from build123d import *

# Parameters (mm, degrees)
BOSS_EXTRUDE1_DEPTH            = 15
SKETCH11_W                     = 2.25
SKETCH11_H                     = 12.7
M4_CLEARANCE_HOLE5_AT_2_COUNT  = 2
M4_CLEARANCE_HOLE5_AT_2_PITCH  = 35
SKETCH13_W                     = 3.75
SKETCH13_H                     = 29.3
F_6_0MM_DOWEL_HOLE1_AT_2_COUNT = 2
F_6_0MM_DOWEL_HOLE1_AT_2_PITCH = 35
FILLET1_R                      = 6.35


with BuildPart() as part:
    # Sketch1 → Boss-Extrude1 (new body)
    with BuildSketch(Plane(origin=(0, 0, 0), x_dir=(1, 0, 0), z_dir=(0, 1, 0))):
        Polygon((0, 0), (0, 42), (22, 20), (44, 42), (44, 0), align=None)
    extrude(amount=BOSS_EXTRUDE1_DEPTH)

    # Sketch11 → M4 Clearance Hole5 (revolve, cut)
    with BuildSketch(Plane(origin=(39.5, 7.5, -12.7), x_dir=(0, 1, 0), z_dir=(1, 0, 0))):
        with Locations((1.125, 6.35)):
            Rectangle(SKETCH11_W, SKETCH11_H)
    m4_clearance_hole5 = revolve(axis=Axis((39.5, 7.5, -19.05), (0, 0, 1)), mode=Mode.SUBTRACT)

    # M4 Clearance Hole5 at 2: M4 Clearance Hole5 ×2
    with Locations(*[(-i * M4_CLEARANCE_HOLE5_AT_2_PITCH, 0, 0) for i in range(1, M4_CLEARANCE_HOLE5_AT_2_COUNT)]):
        add(m4_clearance_hole5, mode=Mode.SUBTRACT)

    # Sketch13 → Ø6.0mm Dowel Hole1 (revolve, cut)
    with BuildSketch(Plane(origin=(39.5, 7.5, -12.7), x_dir=(0, -1, 0), z_dir=(1, 0, 0))):
        with Locations((1.875, 14.65)):
            Rectangle(SKETCH13_W, SKETCH13_H)
    f_6_0mm_dowel_hole1 = revolve(axis=Axis((39.5, 7.5, -6.35), (0, 0, -1)), mode=Mode.SUBTRACT)

    # Ø6.0mm Dowel Hole1 at 2: Ø6.0mm Dowel Hole1 ×2
    with Locations(*[(-i * F_6_0MM_DOWEL_HOLE1_AT_2_PITCH, 0, 0) for i in range(1, F_6_0MM_DOWEL_HOLE1_AT_2_COUNT)]):
        add(f_6_0mm_dowel_hole1, mode=Mode.SUBTRACT)

    # Fillet1
    fillet1_edges = [part.edges().sort_by_distance(p)[0] for p in [
        (22, 7.5, -20),
    ]]
    fillet(fillet1_edges, radius=FILLET1_R)


solid = part.part
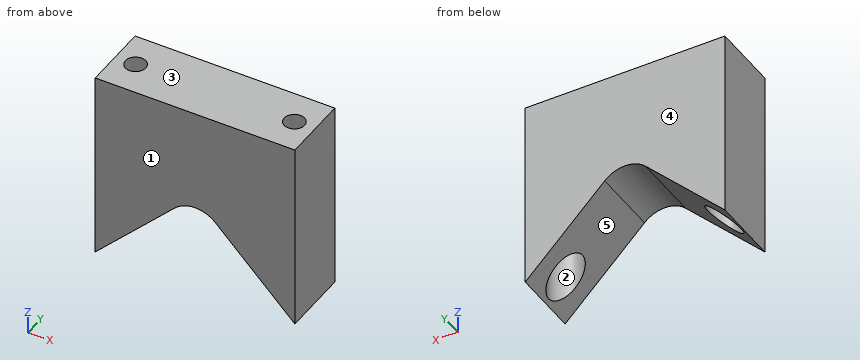
Verification items for the finished model (mm, model axes). Face numbers are marked on the shaded views. A direction names the side the tool comes from. Coordinates: 2 decimals unless noted, no trailing zeros. Write each loop counter-clockwise with the first axis right and the second up, starting at its lowest first coordinate (ties: lowest second). Pieces come first, ordered by that corner, then holes. Notation, with made-up numbers: (42.5, 68.5) -> (98.5, 68.5) arc R16 ccw to (98.5, 86.5) -> close; hole circle Ø9 at (60.5, 80). An arc over 180 degrees is marked (long way). One line per item, written item: value. Start each with the question number.
Q1. Thickness scan on L1, parallel to X at y = 10.5, z = -22; L2, parallel to X at y = 7.5, z = -22; L3, parallel to Y at x = 4.5, z = -32.75. Record the ranges inside material, lowest first. Write a range as from..to.
Q2. Cross-section at A-A on z = -31.5. Enter the section's corners in (x, y), and give its area (3 significant figures).
Q3. Cross-section at B-B on y = 7.5. Enter the section's corners in (x, z), and give its area (3 significant figures).
Q4. Cross-section at D-D on z = -14. Enter the section's corners in (x, y).
Q5. Access from +Z, -Z, +X, -X, +Y, -Y to the whole of each face (thin tool, end or side, straight path). Record for the marked faces 4 and 5.
Q6. Mould release check, pull along Y, two halves, no side actions. Record for the marked faces 1, 2 and 3: pulls with the +Y half, pulls with the -Y half, needs draft (parallel to the pull), parting line crosses it, or undercut.
Q7. Cross-section at C-C on x = 4.5. Enter the section's corners in (y, z), and give its area (3 significant figures).
Q8. Go/stop test with flat-tipped pins: P1, Ø2, axis at x = 40.5, y = 7.5, coming from the -Z side; P2, Ø6, axis at x = 4.5, y = 7.5, coming from the +Z side; P3, Ø3, axis at x = 13, y = 9.5, coming from the -Z side; P4, Ø3, axis at x = 25, y = 11, coming from the -Z side. Record where each tip stops, or that it passes through.
Checked values:
1. L1: x = 0..2.25, 6.75..37.25, 41.75..44
1. L2: x = 0..0.75, 8.25..35.75, 43.25..44
1. L3: y = 0..3.75, 11.25..15
2. outline: (0, 0) -> (10.5, 0) -> (10.5, 15) -> (0, 15) -> close; (33.5, 0) -> (44, 0) -> (44, 15) -> (33.5, 15) -> close; hole circle Ø7.5 at (4.5, 7.5); hole circle Ø7.5 at (39.5, 7.5)
2. area: 227 mm²
3. outline: (0, -42) -> (0.75, -41.25) -> (0.75, -12.7) -> (2.25, -12.7) -> (2.25, 0) -> (0, 0) -> close; (6.75, -12.7) -> (8.25, -12.7) -> (8.25, -33.75) -> (17.51, -24.49) arc R6.35 cw to (26.49, -24.49) -> (35.75, -33.75) -> (35.75, -12.7) -> (37.25, -12.7) -> (37.25, 0) -> (6.75, 0) -> close; (41.75, -12.7) -> (43.25, -12.7) -> (43.25, -41.25) -> (44, -42) -> (44, 0) -> (41.75, 0) -> close
3. area: 886 mm²
4. outline: (0, 0) -> (44, 0) -> (44, 15) -> (0, 15) -> close; hole circle Ø7.5 at (4.5, 7.5); hole circle Ø7.5 at (39.5, 7.5)
5. face 4: +Z, -Z, +X, -X, +Y
5. face 5: -Z, +Y, -Y
6. face 1: pulls with the -Y half
6. face 2: undercut
6. face 3: needs draft
7. outline: (0, -37.5) -> (3.75, -37.5) -> (3.75, -12.7) -> (5.25, -12.7) -> (5.25, 0) -> (0, 0) -> close; (9.75, -12.7) -> (11.25, -12.7) -> (11.25, -37.5) -> (15, -37.5) -> (15, 0) -> (9.75, 0) -> close
7. area: 319 mm²
8. P1: passes through
8. P2: stops at z = 0
8. P3: stops at z = -30.5
8. P4: stops at z = -24.5
